For this review, take the finished solid that the model builds, in its own axes (mm). Face numbers are marked on the shaded views. Give positions to 0.01 mm unless a question says otherwise; leave off trailing zeros. Order: outer loops, then holes, each group sorted by start corner. A loop starts at its lowest first (then second) coordinate and runs counter-clockwise, first axis right, second up. Notation, with made-up numbers: (-5.5, 43.5) - (1.5, 43.5) arc R18 ccw to (1.5, 54.5) - close; hole circle Ø10 at (27, 36). An arc over 180 degrees is marked (long way). Use a Markdown table: item, result. Add a question column.
1) We need section C-C on z = 79.5. Write out the cut boundary in (x, y) (3 decimals), then the cut area to 3 significant figures.
2) Clearance check with flat-ended pins moving along their axes: P1, Ø1.5, axis at x = -5.5, y = -265, coming from the +Z side; P2, Ø6, axis at x = 32, y = -394, coming from the +Z side; P3, Ø2, axis at x = 5.5, z = -15, coming from the -Y side (3 decimals). State where each tip first meets the part, or that it passes through.
3) We need section A-A on z = -9. Write out the cut boundary in (x, y) (3 decimals).
4) We need section D-D on y = -391. Write out the cut boundary in (x, z) (3 decimals).
5) Mouldability with a two-part tool opening along Y and no side actions: class the marked faces 1, 2 and 3 as released by +Y, released by -Y, zero draft, split by the parting line, or undercut.
6) Wall thickness on L1, parallel to Y at x = 37, z = 47.5 (3 decimals); L2, parallel to Y at x = -26.5, z = 100.5 (3 decimals); L3, parallel to Z at x = -2, y = -24.5 (3 decimals): over which ranges is each line inside the solid? List them lowest first.
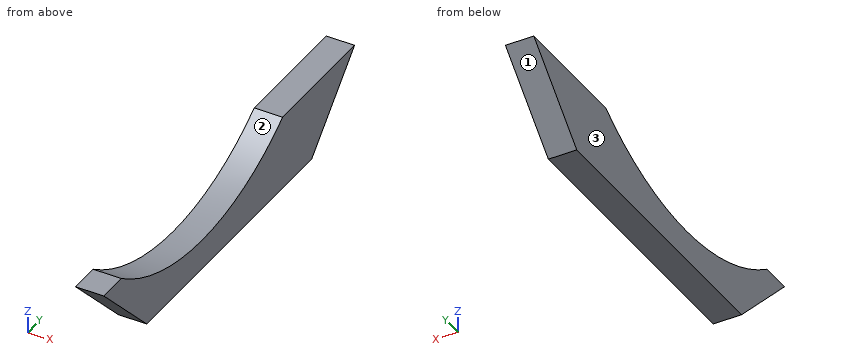
```python
from build123d import *

# Parameters (mm, degrees)
F0_W     = 88.9
F0_H     = 234.95
F1_DEPTH = 685.8
F2_SIZE  = 234.94999
F3_SIZE  = 234.94999
F5_D     = 1524


# Not quite as in the source:
# - a fillet or chamfer is up to 0.001 mm smaller than in the source, because OpenCascade refuses the exact size


with BuildPart() as f1:
    # F0 (on Front) → F1 (new body, symmetric)
    with BuildSketch(Plane.XZ):
        Rectangle(F0_W, F0_H)
    extrude(amount=F1_DEPTH, both=True)

    # F2 (size 234.95 in the source; OpenCascade refuses exactly that, so slightly less here)
    f2_edges = [f1.edges().sort_by_distance(p)[0] for p in [
        (0, -685.8, -117.475),
    ]]
    chamfer(f2_edges, length=F2_SIZE)

    # F3 (size 234.95 in the source; OpenCascade refuses exactly that, so slightly less here)
    f3_edges = [f1.edges().sort_by_distance(p)[0] for p in [
        (0, 685.8, -117.475),
    ]]
    chamfer(f3_edges, length=F3_SIZE)

    # F5 (through all)
    with Locations(Plane(origin=(-44.45, 0, 0), x_dir=(0, -1, 0), z_dir=(-1, 0, 0))):
        with Locations((148.8177627325, 738.7712001801)):
            Hole(F5_D / 2)


solid = f1.part
```
Checked values:
| question | item | result |
|---|---|---|
| 1 | outline | (-44.45, -647.825) - (44.45, -647.825) - (44.45, -530.924) - (-44.45, -530.924) - close; (-44.45, 233.289) - (44.45, 233.289) - (44.45, 647.825) - (-44.45, 647.825) - close |
| 1 | area | 47,200 mm² |
| 2 | P1 | z = -14.2 |
| 2 | P2 | z = 18.32 |
| 2 | P3 | y = -554.325 |
| 3 | outline | (-44.45, -559.325) - (44.45, -559.325) - (44.45, -295.386) - (-44.45, -295.386) - close; (-44.45, -2.25) - (44.45, -2.25) - (44.45, 559.325) - (-44.45, 559.325) - close |
| 4 | outline | (-44.45, -117.475) - (44.45, -117.475) - (44.45, 16.281) - (-44.45, 16.281) - close |
| 5 | face 1 | released by +Y |
| 5 | face 2 | undercut |
| 5 | face 3 | zero draft |
| 6 | L1 | -615.825 to -469.424, 171.788 to 615.825 |
| 6 | L2 | -668.825 to -565.056, 267.42 to 668.825 |
| 6 | L3 | -117.475 to -13.019 |
